Autodesk Inventor part; units mm, degrees
ref_plane "YZ Plane" through (0, 0, 0) normal (1, 0, 0) x (0, 1, 0)
ref_plane "XZ Plane" through (0, 0, 0) normal (0, 1, 0) x (-1, 0, 0)
ref_plane "XY Plane" through (0, 0, 0) normal (0, 0, 1) x (1, 0, 0)
sketch "Boceto1" plane through (0, 0, 0) normal (0, 1, 0) x (-1, 0, 0)
  line L0 (-7.5247, -31.1664) -> (-7.5247, 0.8336)
  line L1 (-7.5247, 0.8336) -> (-9.5247, 0.8336)
  line L2 (-9.5247, 0.8336) -> (-9.5247, -29.1664)
  line L3 (-7.5247, -31.1664) -> (-39.5247, -31.1664)
  line L4 (-39.5247, -31.1664) -> (-39.5247, -29.1664)
  line L5 (-39.5247, -29.1664) -> (-9.5247, -29.1664)
  dimension "d46" = 32
  dimension "d47" = 2
  dimension "d48" = 30
  dimension "d49" = 32
extrude "Extrusion9" add sketch "Boceto1" along normal blind 14
fillet "Fillet1" radius 0.5 1 edges at (9.5247, 7, -29.1664)
fillet "Fillet2" radius 2.5 1 edges at (7.5247, 7, -31.1664)
sketch "Sketch6" plane through (9.5247, 0, 0.8336) normal (1, 0, 0) x (0, 0, -1)
  circle A0 centre (8.5, 7) radius 2
  line L0 (30, 0) -> (30, 14)
  line L1 (0, 0) -> (29.5, 0)
  dimension "d54" = 4
  dimension "d55" = 21.5
  dimension "d56" = 7
sketch "Sketch7" plane through (39.5247, 0, -29.1664) normal (0, 0, 1) x (1, 0, 0)
  circle A0 centre (-8.5, 7) radius 2
  line L0 (-29.5, 0) -> (0, 0)
  line L1 (-30, 14) -> (-30, 0)
  dimension "d57" = 4
  dimension "d58" = 7
  dimension "d59" = 21.5
extrude "Extrusion10" cut sketch "Sketch6" against normal blind 10
extrude "Extrusion11" cut sketch "Sketch7" against normal blind 10
properties part number "Esquina de bandeja" material "Aluminum 1100-H14"
Can you work these out from the model? Positions are in its coordinate system, mm. A direction names the side the tool comes from. Give positions to 0.01 mm unless a question says otherwise; leave off trailing zeros. Order: outer loops, then holes, each group sorted by start corner. A loop starts at its lowest first (then second) coordinate and runs counter-clockwise, first axis right, second up. Notation, with made-up numbers: M 58.25,73.5 L 106.25,73.5 A20 cw 106.25,80.5 Z; hole C 72.5,66.5 d1. An arc over 180 degrees is marked long. One line per item, written item: value.
1) For P1, Ø7, axis at x = 19, y = 9.5, coming from the +Z side; P2, Ø7, axis at y = 9, z = -15, coming from the +X side, each with a flat end and sliding along its axis, tell me the tip position at first contact or that it passes through.
Answer sheet:
P1: stops at z = -29.17
P2: stops at x = 9.52
2) I want a section at C-C, the plane z = -7. List the corners of the cut face in (x, y) for me.
Answer sheet:
outline: M 7.52,0 L 9.52,0 L 9.52,5.11 L 7.52,5.11 Z; M 7.52,8.89 L 9.52,8.89 L 9.52,14 L 7.52,14 Z
3) We'd pull the mould along Z, two halves only. Please class faces 1 (the face through (8.539, 8.686, -8.742)), 2 (the face through (7.525, 7, -14)), 3 (the face through (8.276, 7.098, -30.453)): released by +Z, released by -Z, zero draft, split by the parting line, or undercut.
Answer sheet:
face 1: undercut
face 2: zero draft
face 3: released by -Z
4) Please list where these lines run through material, in increasing order: line 1 along X through (y, z) = (4.75, -12); line 2 along Z through (x, y) = (10.5, 11.25).
Answer sheet:
line 1: x = 7.52 to 9.52
line 2: z = -31.17 to -29.17
5) I want a section at B-B, the plane y = 3.5. List the corners of the cut face in (x, z) for me, plus the area to 3 significant figures.
Answer sheet:
outline: M 7.52,-28.67 A2.5 ccw 10.02,-31.17 L 39.52,-31.17 L 39.52,-29.17 L 10.02,-29.17 A0.5 cw 9.52,-28.67 L 9.52,0.83 L 7.52,0.83 Z
area: 123 mm^2
6) I want a section at D-D, the plane x = 25. List the corners of the cut face in (y, z) for me, plus the area to 3 significant figures.
Answer sheet:
outline: M 0,-31.17 L 14,-31.17 L 14,-29.17 L 0,-29.17 Z
area: 28.0 mm^2
7) I want a section at A-A, the plane y = 7. List the corners of the cut face in (x, z) for me.
Answer sheet:
outline: M 7.52,-28.67 A2.5 ccw 10.02,-31.17 L 29.02,-31.17 L 29.02,-29.17 L 10.02,-29.17 A0.5 cw 9.52,-28.67 L 9.52,-9.67 L 7.52,-9.67 Z; M 7.52,-5.67 L 9.52,-5.67 L 9.52,0.83 L 7.52,0.83 Z; M 33.02,-31.17 L 39.52,-31.17 L 39.52,-29.17 L 33.02,-29.17 Z
8) On a 3-axis mill with a long thin cutter (end or side, diameter ignored), from which of +Z, -Z, +X, -X, +Y, -Y can I reach the whole of each face in a straight line? I mean faces 4 (the face through (29.55, 8.35, -30.15)), 5 (the face through (9.525, 7, -14)). Say none if no direction works.
Answer sheet:
face 4: +Z, -Z
face 5: +Z, +X, +Y, -Y
